from build123d import *

# Parameters (mm, degrees)
F1_DEPTH  = 37
F2_W      = 22
F2_H      = 22
F3_DEPTH  = 260
F4_W      = 37
F4_H      = 62
F5_DEPTH  = 30
F6_W      = 22
F6_H      = 22
F7_DEPTH  = 380
F8_W      = 20
F8_H      = 5
F9_DEPTH  = 25
F10_R     = 3
F11_DEPTH = 37.001
F13_R     = 3
F14_DEPTH = 17


with BuildPart() as f1:
    # F0 (on Front) → F1 (new body)
    with BuildSketch(Plane.XZ):
        Polygon((0, -280), (0, 0), (-62, 0), (-62, -218), (-440, -218), (-440, -280), align=None)
    extrude(amount=F1_DEPTH)

    # F2 (on face) → F3 (cut)
    with BuildSketch(Plane.XY):
        with Locations((-31, -26)):
            Rectangle(F2_W, F2_H)
    extrude(amount=-F3_DEPTH, mode=Mode.SUBTRACT)

    # F4 (on face) → F5 (join)
    with BuildSketch(Plane.YZ):
        with Locations((-18.5, -249)):
            Rectangle(F4_W, F4_H)
    extrude(amount=F5_DEPTH)

    # F6 (on face) → F7 (cut)
    with BuildSketch(Plane.YZ.offset(-42)):
        with Locations((-26, -249)):
            Rectangle(F6_W, F6_H)
    extrude(amount=-F7_DEPTH, mode=Mode.SUBTRACT)

    # F8 (on face) → F9 (cut)
    with BuildSketch(Plane.XY.offset(-218)):
        with Locations((-370, -34.5)):
            Rectangle(F8_W, F8_H)
    extrude(amount=-F9_DEPTH, mode=Mode.SUBTRACT)

    # F10 (on face) → F11 (cut, through all)
    with BuildSketch(Plane.XZ.offset(37)):
        with Locations((-52, -10)):
            Circle(F10_R)
        with Locations((-10, -10)):
            Circle(F10_R)
        with Locations((-52, -80)):
            Circle(F10_R)
        with Locations((-10, -80)):
            Circle(F10_R)
        with Locations((-52, -138)):
            Circle(F10_R)
        with Locations((-10, -138)):
            Circle(F10_R)
        with Locations((-52, -218)):
            Circle(F10_R)
        with Locations((-10, -218)):
            Circle(F10_R)
        with Locations((10, -248)):
            Circle(F10_R)
        with Locations((-232, -270)):
            Circle(F10_R)
        with Locations((-232, -228)):
            Circle(F10_R)
        with Locations((-430, -248)):
            Circle(F10_R)
    extrude(amount=-F11_DEPTH, mode=Mode.SUBTRACT)

    # F13 (on face) → F14 (cut)
    with BuildSketch(Plane.XY.offset(-218)):
        with Locations((-415, -27)):
            Circle(F13_R)
        with Locations((-325, -27)):
            Circle(F13_R)
    extrude(amount=-F14_DEPTH, mode=Mode.SUBTRACT)


solid = f1.part
Check sheet for the modelled part. Datum: model origin and axes. Units: mm. A direction names the side the tool comes from. Give positions to 0.01 mm unless a question says otherwise; leave off trailing zeros. Write each loop counter-clockwise with the first axis right and the second up, starting at its lowest first coordinate (ties: lowest second). Pieces come first, ordered by that corner, then holes. Notation, with made-up numbers: (75, 88) -> (128, 88) arc R25 ccw to (128, 106) -> close; hole circle Ø10 at (-18.75, 54). An arc over 180 degrees is marked (long way). One line per item, written item: value. Start each with the question number.
Item 1: Gauge pin test, flat ends, axial feed: pin 1 (11 mm diameter, centred on y = -31.5, z = -187.5, fed in from -X); pin 2 (12 mm diameter, centred on x = -257, y = -5, fed in from +Z); pin 3 (5 mm diameter, centred on y = -19, z = -126, fed in from +X). Record the tip position at first contact, or that the pin passes through.
Item 2: Section check C-C on x = -191. Record the cut outline in (y, z).
Item 3: Section check D-D on x = -34.5. Record the cut outline in (y, z).
Item 4: Section check A-A on y = -8. State how many separate pieces and enclosed holes the cut face has, then the cut area to 3 significant figures.
Item 5: Tool access check on faces 1 (the flat face through (-248, -18, -218)), 2 (the flat face through (-370, -32, -228)), 3 (the flat face through (0, -18, -111)), 4 (the flat face through (-31, -14, 0)), 5 (the flat face through (-229, -26, -238)). Record the directions out of +Z, -Z, +X, -X, +Y, -Y that give a thin tool (end or side, any length) a straight path to the whole face; none if there is none.
Item 6: Material ranges on probe 1 along Z at (x, y) = (-10, -15.5); probe 2 along X at (y, z) = (-18, -138); probe 3 along Z at (x, y) = (-225, -20.5), recorded low to high. Write a range as from..to.
Item 7: Section check B-B on z = -49. Record the cut outline in (x, y), then the cut area to 3 significant figures.
Item 8: Draft check along X on faces 6 (the flat face through (-422, -26, -249)), 7 (the flat face through (30, -19, -249)), 8 (the flat face through (-208, -19, -280)). Enter one of: +X half, -X half, draft (parallel to the pull), parting line (faces both ways), or undercut.
Results list:
1. pin 1: x = -62
1. pin 2: z = -218
1. pin 3: x = 0
2. outline: (-37, -280) -> (0, -280) -> (0, -218) -> (-37, -218) -> (-37, -238) -> (-15, -238) -> (-15, -260) -> (-37, -260) -> close
3. outline: (-37, -280) -> (0, -280) -> (0, 0) -> (-15, 0) -> (-15, -260) -> (-37, -260) -> close
4. separate pieces: 1
4. enclosed holes: 12
4. area: 42,300 mm²
5. face 1: +Z, -X, +Y, -Y
5. face 2: +Z, -Y
5. face 3: +Z, +X, +Y, -Y
5. face 4: +Z, +X, -X, +Y, -Y
5. face 5: -Y
6. probe 1: -280..-221, -215..-141, -135..-83, -77..-13, -7..0
6. probe 2: -62..-55, -49..-42, -20..-13, -7..0
6. probe 3: -280..-260, -238..-218
7. outline: (-62, -37) -> (-42, -37) -> (-42, -15) -> (-20, -15) -> (-20, -37) -> (0, -37) -> (0, 0) -> (-62, 0) -> close
7. area: 1,810 mm²
8. face 6: undercut
8. face 7: +X half
8. face 8: draft
